CAD build for the part. Positions are in the model's coordinates, mm. A direction names the side the tool comes from. Coordinates: 2 decimals unless noted, no trailing zeros. Write each loop counter-clockwise with the first axis right and the second up, starting at its lowest first coordinate (ties: lowest second). Pieces come first, ordered by that corner, then holes. Notation, with made-up numbers: M 67.5,-36 L 81.5,-36 A20 cw 81.5,0 Z; hole C 37.25,17 d1. An arc over 180 degrees is marked long. Put each result on its own line as item: value. Start each with the question number.
```python
from build123d import *

# Parameters (mm, degrees)
SKETCH_W        = 130
SKETCH_H        = 32
PAD_DEPTH       = 8
SKETCH001_R     = 2.35
SKETCH001_R_2   = 2.75
POCKET_DEPTH    = 8.001
SKETCH003_R     = 4.6
POCKET001_DEPTH = 5
SKETCH002_R     = 2.25
POCKET002_DEPTH = 8.001
CHAMFER_SIZE    = 2
FILLET_R        = 5


with BuildPart() as part:
    # Sketch → Pad (new body)
    with BuildSketch(Plane.XY):
        Rectangle(SKETCH_W, SKETCH_H)
    extrude(amount=PAD_DEPTH)

    # Sketch001 → Pocket (cut, through all)
    with BuildSketch(Plane.XY.offset(8)):
        with Locations((-35, 9)):
            Circle(SKETCH001_R)
        with Locations((-58.997728, -9)):
            Circle(SKETCH001_R)
        with Locations((-59, 9)):
            Circle(SKETCH001_R)
        with Locations((35, 9)):
            Circle(SKETCH001_R)
        with Locations((59, -9)):
            Circle(SKETCH001_R)
        with Locations((59, 9)):
            Circle(SKETCH001_R)
        with Locations((-47, 9)):
            Circle(SKETCH001_R_2)
        with Locations((-47, -11)):
            Circle(SKETCH001_R_2)
        with Locations((47, 9)):
            Circle(SKETCH001_R_2)
        with Locations((47, -11)):
            Circle(SKETCH001_R_2)
        with Locations((-21, 0)):
            Circle(SKETCH001_R_2)
        with Locations((21, 0)):
            Circle(SKETCH001_R_2)
        with Locations((-35, -9)):
            Circle(SKETCH001_R)
        with Locations((35, -9)):
            Circle(SKETCH001_R)
    extrude(amount=-POCKET_DEPTH, mode=Mode.SUBTRACT)

    # Sketch003 → Pocket001 (cut)
    with BuildSketch(Plane.XY.offset(8)):
        with Locations((-47, 9)):
            Circle(SKETCH003_R)
        with Locations((47, -11)):
            Circle(SKETCH003_R)
        with Locations((47, 9)):
            Circle(SKETCH003_R)
        with Locations((-47, -11)):
            Circle(SKETCH003_R)
    extrude(amount=-POCKET001_DEPTH, mode=Mode.SUBTRACT)

    # Sketch002 → Pocket002 (cut, through all)
    with BuildSketch(Plane.XY.offset(8)):
        with Locations((-10, 10)):
            Circle(SKETCH002_R)
        with Locations((-10, 0)):
            Circle(SKETCH002_R)
        with Locations((10, 10)):
            Circle(SKETCH002_R)
        with Locations((10, 0)):
            Circle(SKETCH002_R)
        with Locations((0, 10)):
            Circle(SKETCH002_R)
        Circle(SKETCH002_R)
        with Locations((0, -10)):
            Circle(SKETCH002_R)
        with Locations((-10, -10)):
            Circle(SKETCH002_R)
        with Locations((10, -10)):
            Circle(SKETCH002_R)
        with Locations((-20, 10)):
            Circle(SKETCH002_R)
        with Locations((20, 10)):
            Circle(SKETCH002_R)
        with Locations((20, -10)):
            Circle(SKETCH002_R)
        with Locations((-20, -10)):
            Circle(SKETCH002_R)
    extrude(amount=-POCKET002_DEPTH, mode=Mode.SUBTRACT)

    # Chamfer
    chamfer_edges = [part.edges().sort_by_distance(p)[0] for p in [
        (0, 16, 0),
    ]]
    chamfer(chamfer_edges, length=CHAMFER_SIZE)

    # Fillet
    fillet_edges = [part.edges().sort_by_distance(p)[0] for p in [
        (-65, 16, 5),
        (65, 16, 5),
        (-65, -16, 4),
        (65, -16, 4),
    ]]
    fillet(fillet_edges, radius=FILLET_R)


solid = part.part
```
(1) Drill centre lines: line 1 (Y direction, x = 10, z = 3.75); line 2 (Y direction, x = 59, z = 3.75); line 3 (Y direction, x = 47, z = 1.95). Where is each one in solid material? Low to high. Write a range as [from, to].
(2) Slice it at A-A, the plane x = -10. Write the cut outline in (y, z), then the cut area to 3 significant figures.
(3) Slice it at C-C, the plane x = 21. Write the cut outline in (y, z), then the cut area to 3 significant figures.
(4) Slice it at B-B, the plane x = -47. Write the cut outline in (y, z), then the cut area to 3 significant figures.
(5) Two-plate mould, pull along Y, no slides. Class faces 3 (the face through (63, -15, 4)), 4 (the face through (60.084, -11.085, 4.056)), 5 (the face through (-1, 4, 8)): +Y half, -Y half, draft (parallel to the pull), parting line (faces both ways), or undercut.
(6) Which spindle directions (+Z, -Z, +X, -X, +Y, -Y) get a long thin tool onto all of the face, cutting with end or side? Do faces 1 (the face through (60.084, 6.915, 4.056)), 2 (the face through (-42.75, -12.76, 5.54)). Say none if no direction does.
(7) Drop a flat-ended pin along its axis: pin 1 (7.5 mm diameter, centred on x = -47, y = -11, fed in from +Z). Give the stop position or say it passes through.
Result set:
1. line 1: y = [-16, -12.25], [-7.75, -2.25], [2.25, 7.75], [12.25, 16]
1. line 2: y = [-16, -11.35], [-6.65, 6.65], [11.35, 16]
1. line 3: y = [-16, -13.75], [-8.25, 6.25], [11.75, 15.95]
2. outline: M -16,0 L -12.25,0 L -12.25,8 L -16,8 Z; M -7.75,0 L -2.25,0 L -2.25,8 L -7.75,8 Z; M 2.25,0 L 7.75,0 L 7.75,8 L 2.25,8 Z; M 12.25,0 L 14,0 L 16,2 L 16,8 L 12.25,8 Z
2. area: 146 mm^2
3. outline: M -16,0 L -12.02,0 L -12.02,8 L -16,8 Z; M -7.98,0 L -2.75,0 L -2.75,8 L -7.98,8 Z; M 2.75,0 L 7.98,0 L 7.98,8 L 2.75,8 Z; M 12.02,0 L 14,0 L 16,2 L 16,8 L 12.02,8 Z
3. area: 146 mm^2
4. outline: M -16,0 L -13.75,0 L -13.75,3 L -15.6,3 L -15.6,8 L -16,8 Z; M -8.25,0 L 6.25,0 L 6.25,3 L 4.4,3 L 4.4,8 L -6.4,8 L -6.4,3 L -8.25,3 Z; M 11.75,0 L 14,0 L 16,2 L 16,8 L 13.6,8 L 13.6,3 L 11.75,3 Z
4. area: 129 mm^2
5. face 3: -Y half
5. face 4: undercut
5. face 5: draft
6. face 1: +Z, -Z
6. face 2: +Z
7. pin 1: stops at z = 3
